Input: dimensioned drawing with shaded views. Units: mm. Origin: part minimum x, y, z. Give positions to 0.01 mm unless a question says otherwise; leave off trailing zeros. Order: outer loops, then holes, each group sorted by start corner. A loop starts at its lowest first (then second) coordinate and runs counter-clockwise, first axis right, second up. Notation, with made-up numbers: (-19, -27) -> (-15, -27) arc R18 ccw to (-15, 4) -> close; hole circle Ø11 at (37.5, -29). An arc over 180 degrees is marked (long way). Use CSV: the item, a comma, the result in double quotes.
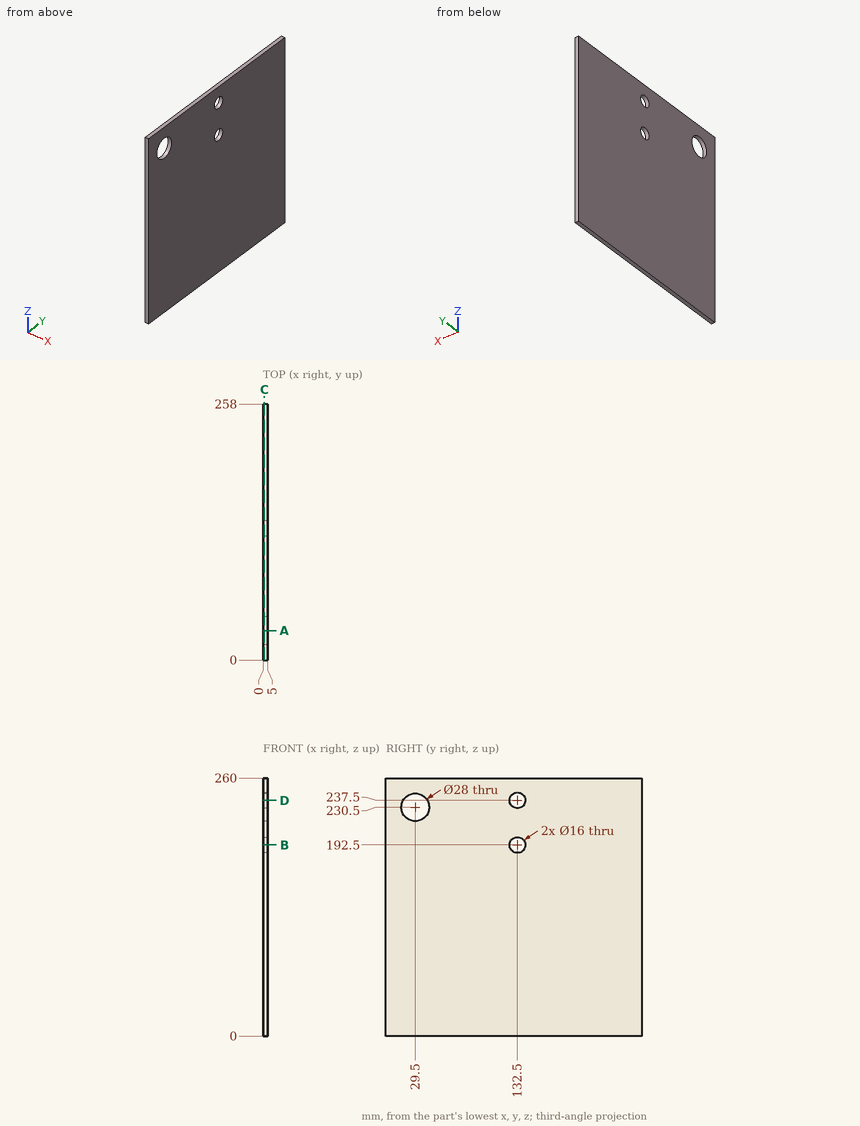
1. Ray query, line 1 along Z through (x, y) = (0.85, 30.5); line 2 along Y through (x, z) = (2.15, 230.5); line 3 along Y through (x, z) = (3.05, 192.5). Return the intervals inside material, ascending.
Answer below:
line 1,"z = 0 to 216.54, 244.46 to 260"
line 2,"y = 0 to 15.5, 43.5 to 128.63, 136.37 to 258"
line 3,"y = 0 to 124.5, 140.5 to 258"
2. Section query C-C on x = 1.35. Return loops of the section in (y, z), plus the area to 3 significant figures.
Answer below:
outline,"(0, 0) -> (258, 0) -> (258, 260) -> (0, 260) -> close; hole circle Ø28 at (29.5, 230.5); hole circle Ø16 at (132.5, 192.5); hole circle Ø16 at (132.5, 237.5)"
area,"66,100 mm²"
3. Section query A-A on y = 29.5. Return loops of the section in (x, z), plus the area to 3 significant figures.
Answer below:
outline,"(0, 0) -> (5, 0) -> (5, 216.5) -> (0, 216.5) -> close; (0, 244.5) -> (5, 244.5) -> (5, 260) -> (0, 260) -> close"
area,"1,160 mm²"
4. Section query D-D on z = 237.5. Return loops of the section in (x, y), plus the area to 3 significant figures.
Answer below:
outline,"(0, 0) -> (5, 0) -> (5, 17.38) -> (0, 17.38) -> close; (0, 41.62) -> (5, 41.62) -> (5, 124.5) -> (0, 124.5) -> close; (0, 140.5) -> (5, 140.5) -> (5, 258) -> (0, 258) -> close"
area,"1,090 mm²"
5. Section query B-B on z = 192.5. Return loops of the section in (x, y), plus the area to 3 significant figures.
Answer below:
outline,"(0, 0) -> (5, 0) -> (5, 124.5) -> (0, 124.5) -> close; (0, 140.5) -> (5, 140.5) -> (5, 258) -> (0, 258) -> close"
area,"1,210 mm²"
